Check sheet for the drawn part. Datum: minimum x, y, z corner. Units: mm. Give positions to 0.01 mm unless a question says otherwise; leave off trailing zeros. Write each loop counter-clockwise with the first axis right and the second up, starting at its lowest first coordinate (ties: lowest second). Pieces come first, ordered by that corner, then holes.
(1) Cross-section at A-A (x = 31.95). Record the boundary of the cut face in (y, z).
(2) Thickness scan on line 1 along Y through (x, z) = (3.05, 1.05); line 2 along X through (y, z) = (13, 1.5) (1 decimal); line 3 along Y through (x, z) = (27, 0.65). Record the ranges inside material, lowest first.
(3) Cross-section at C-C (y = 15). Record the boundary of the cut face in (x, z) (1 decimal).
(4) Cross-section at B-B (y = 22.75). Record the boundary of the cut face in (x, z).
(5) Cross-section at D-D (z = 1.3). Count the separate pieces of the cut face and the enclosed holes in it, and give its area (3 significant figures).
(6) Depth check by flat-ended pin: P1, Ø3, axis at x = 31.95, y = 15, coming from the -Z side; P2, Ø2, axis at x = 3.05, y = 26.95, coming from the +Z side. Enter the tip coordinate at first touch or a pass-through.
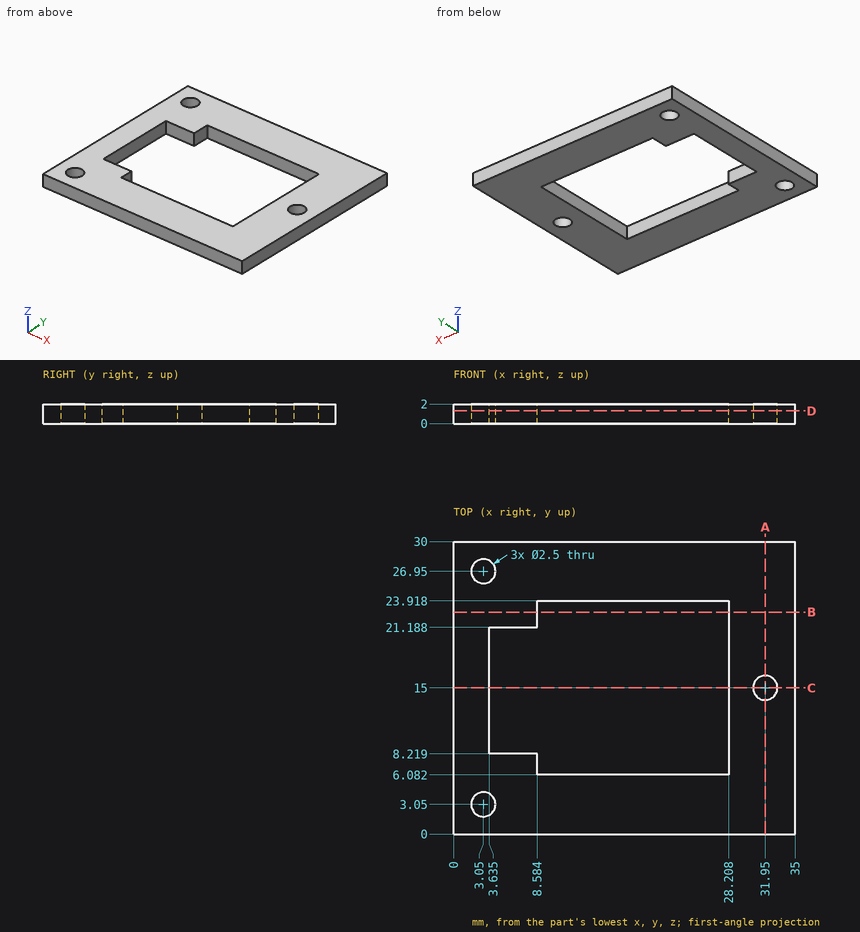
Reply:
1. outline: (0, 0) - (13.75, 0) - (13.75, 2) - (0, 2) - close; (16.25, 0) - (30, 0) - (30, 2) - (16.25, 2) - close
2. line 1: y = 0 to 1.8, 4.3 to 25.7, 28.2 to 30
2. line 2: x = 0 to 3.6, 28.2 to 35
2. line 3: y = 0 to 6.08, 23.92 to 30
3. outline: (0, 0) - (3.6, 0) - (3.6, 2) - (0, 2) - close; (28.2, 0) - (30.7, 0) - (30.7, 2) - (28.2, 2) - close; (33.2, 0) - (35, 0) - (35, 2) - (33.2, 2) - close
4. outline: (0, 0) - (8.58, 0) - (8.58, 2) - (0, 2) - close; (28.21, 0) - (35, 0) - (35, 2) - (28.21, 2) - close
5. separate pieces: 1
5. enclosed holes: 4
5. area: 621 mm2
6. P1: stops at z = 0
6. P2: passes through
